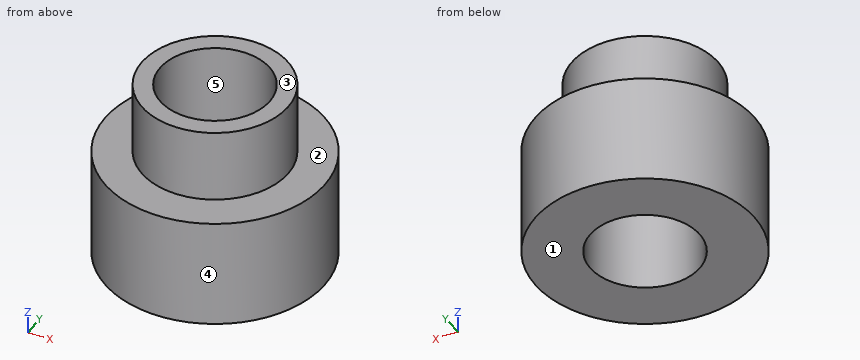
from build123d import *

# Parameters (mm, degrees)
SKETCH_1_R          = 3
EXTRUDE_1_DEPTH     = 3
SKETCH_1_3_R        = 2
EXTRUDE_2_DEPTH     = 5
SKETCH_1_4_R        = 1.5
CUT_EXTRUDE_1_DEPTH = 6


with BuildPart() as part:
    # Sketch 1 → Extrude 1 (new body)
    with BuildSketch(Plane.XY):
        Circle(SKETCH_1_R)
    extrude(amount=EXTRUDE_1_DEPTH)

    # Sketch 1_3 → Extrude 2 (add)
    with BuildSketch(Plane.XY):
        Circle(SKETCH_1_3_R)
    extrude(amount=EXTRUDE_2_DEPTH)

    # Sketch 1_4 → Cut-Extrude 1 (cut, through all)
    with BuildSketch(Plane.XY):
        Circle(SKETCH_1_4_R)
    extrude(amount=CUT_EXTRUDE_1_DEPTH, mode=Mode.SUBTRACT)


solid = part.part
Work out the finished part from the listing and answer in its coordinate system (mm). Face numbers are marked on the shaded views. A direction names the side the tool comes from. Round coordinates to 2 decimals unless told otherwise and drop trailing zeros. Loops run counter-clockwise (first coordinate to the right, second up) from the corner with the lowest first, then second, coordinate; pieces in that order, holes last. Notation, with made-up numbers: (16, 76) - (30, 76) arc R28 cw to (30, 94) - close; hole circle Ø9 at (72.25, 16). An arc over 180 degrees is marked (long way). Use one line per item in the form item = value. Start each with the question number.
(1) Determine the mould class of the marked faces 3, 4 and 5 for opening direction X: +X half, -X half, draft (parallel to the pull), parting line (faces both ways), or undercut.
(2) Find section D-D on x = 1.65. Determine the outline of the cut face in (y, z).
(3) Find section A-A on y = 0. Determine the outline of the cut face in (x, z), and give its area (3 significant figures).
(4) Find section C-C on z = 0.3. Determine the outline of the cut face in (x, y).
(5) Which of the six approach directions +Z, -Z, +X, -X, +Y, -Y give full straight-line access (tool end or side, diameter ignored) to the marked faces 1 and 2?
(6) Consider line 1 (Y direction, x = 0.05, z = 4.2); line 2 (Y direction, x = 0, z = 1.3). Determine where each line is inside the solid, lowest interval first.
(7) A flat-ended cylindrical pin translates along its axis: P1, Ø3, axis at x = 2, z = 0.5, coming from the -Y side. Find the tip coordinate at first contact, or state that the pin passes through.
Answer list:
q1.face_3 = draft
q1.face_4 = parting line
q1.face_5 = undercut
q2.outline = (-2.51, 0) - (2.51, 0) - (2.51, 3) - (1.13, 3) - (1.13, 5) - (-1.13, 5) - (-1.13, 3) - (-2.51, 3) - close
q3.outline = (-3, 0) - (-1.5, 0) - (-1.5, 5) - (-2, 5) - (-2, 3) - (-3, 3) - close; (1.5, 0) - (3, 0) - (3, 3) - (2, 3) - (2, 5) - (1.5, 5) - close
q3.area = 11.0 mm^2
q4.outline = circle Ø6 at (0, 0); hole circle Ø3 at (0, 0)
q5.face_1 = -Z, +X, -X, +Y, -Y
q5.face_2 = +Z
q6.line_1 = -2 to -1.5, 1.5 to 2
q6.line_2 = -3 to -1.5, 1.5 to 3
q7.P1 = -2.96
